Part print with two shaded views. Sizes in mm from the minimum x, y, z corner. Round coordinates to 2 decimals unless told otherwise and drop trailing zeros. Order: outer loops, then holes, each group sorted by start corner. A loop starts at its lowest first (then second) coordinate and runs counter-clockwise, first axis right, second up. Notation, with made-up numbers: M 50.5,-22 L 73.5,-22 A21 ccw 73.5,-5 Z; hole C 2.5,85.5 d4. An arc over 180 degrees is marked long. Answer as a JSON object with one key per item and string values.
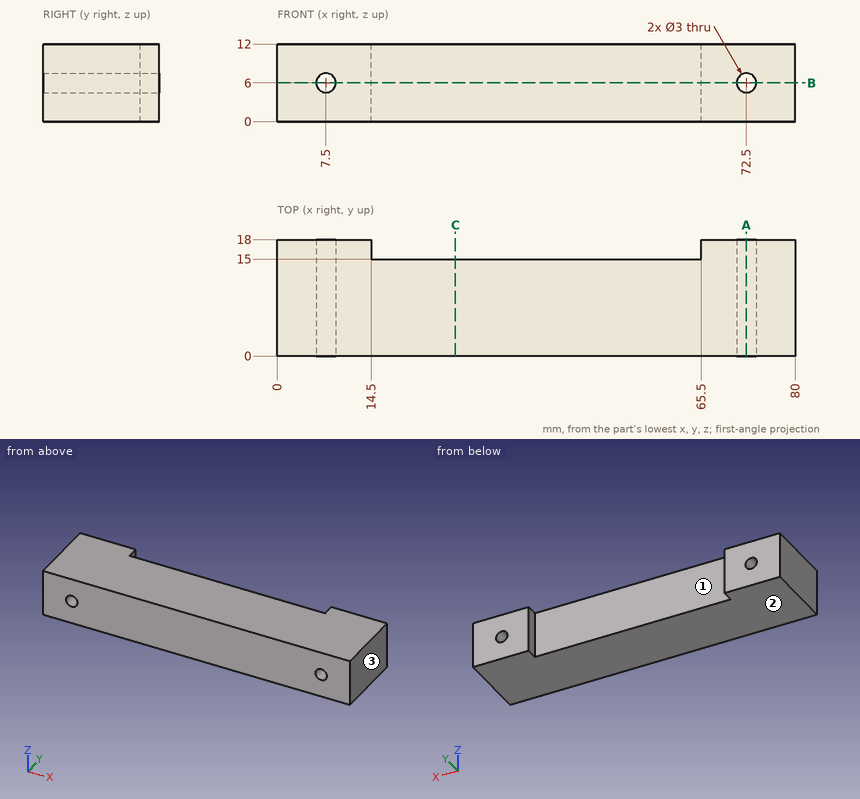
Item 1: Saw through at C-C on x = 27.5. List the corners of the cut face in (y, z).
Worked answers:
{"outline": "M 0,0 L 15,0 L 15,12 L 0,12 Z"}
Item 2: Saw through at A-A on x = 72.5. List the corners of the cut face in (y, z), and give its area (3 significant figures).
Worked answers:
{"outline": "M 0,0 L 18,0 L 18,4.5 L 0,4.5 Z; M 0,7.5 L 18,7.5 L 18,12 L 0,12 Z", "area": "162 mm2"}
Item 3: Wall check: line 1 along X through (y, z) = (14, 6); line 2 along Z through (x, y) = (72.5, 10.5); line 3 along Y through (x, z) = (20.5, 11). Give the ranges that are in metal, low to high. Write a range as [from, to].
Worked answers:
{"line 1": "x = [0, 6], [9, 71], [74, 80]", "line 2": "z = [0, 4.5], [7.5, 12]", "line 3": "y = [0, 15]"}
Item 4: Two-plate mould, pull along X, no slides. Class the marked faces 1, 2 and 3: released by +X, released by -X, zero draft, split by the parting line, or undercut.
Worked answers:
{"face 1": "undercut", "face 2": "zero draft", "face 3": "released by +X"}
Item 5: Saw through at B-B on z = 6. List the corners of the cut face in (x, y).
Worked answers:
{"outline": "M 0,0 L 6,0 L 6,18 L 0,18 Z; M 9,0 L 71,0 L 71,18 L 65.5,18 L 65.5,15 L 14.5,15 L 14.5,18 L 9,18 Z; M 74,0 L 80,0 L 80,18 L 74,18 Z"}
